from build123d import *

# Parameters (mm, degrees)
AUFSATZ_LINEAR_AUSTRAGEN1_DEPTH = 5
DURCHGANGSLOCH_F_R_M41_D        = 4.3
DURCHGANGSLOCH_F_R_M42_D        = 4.3
M4_GEWINDEBOHRUNG1_D            = 3.3
M3_GEWINDEBOHRUNG1_D            = 2.5


with BuildPart() as part:
    # Skizze1 → Aufsatz-Linear austragen1 (new body)
    with BuildSketch(Plane(origin=(0, 0, 0), x_dir=(1, 0, 0), z_dir=(0, 1, 0))):
        Polygon((-9, 15), (-9, -15), (29, -15), (29, 35), (9, 35), (9, 15), align=None)
    extrude(amount=AUFSATZ_LINEAR_AUSTRAGEN1_DEPTH)

    # Durchgangsloch für M41 (through all)
    with Locations(Plane(origin=(0, 5, 0), x_dir=(1, 0, 0), z_dir=(0, 1, 0))):
        with Locations((7, 8), (23, 8), (7, -8), (23, -8)):
            Hole(DURCHGANGSLOCH_F_R_M41_D / 2)

    # Durchgangsloch für M42 (through all)
    with Locations(Plane(origin=(0, 5, 0), x_dir=(1, 0, 0), z_dir=(0, 1, 0))):
        with Locations((-3.5, 8), (-3.5, -8)):
            Hole(DURCHGANGSLOCH_F_R_M42_D / 2)

    # M4 Gewindebohrung1 (through all)
    with Locations(Plane(origin=(0, 5, 0), x_dir=(1, 0, 0), z_dir=(0, 1, 0))):
        with Locations((19, 25)):
            Hole(M4_GEWINDEBOHRUNG1_D / 2)

    # M3 Gewindebohrung1 (through all)
    with Locations(Plane(origin=(0, 5, 0), x_dir=(1, 0, 0), z_dir=(0, 1, 0))):
        with Locations((3, 0)):
            Hole(M3_GEWINDEBOHRUNG1_D / 2)


solid = part.part
Source: CAD feature listing. Evaluate the final solid. Frame: model axes, mm. A direction names the side the tool comes from. Round coordinates to 2 decimals unless told otherwise and drop trailing zeros. Loops run counter-clockwise (first coordinate to the right, second up) from the corner with the lowest first, then second, coordinate; pieces in that order, holes last.
Q1. Section A-A, the plane x = 23. Return loops of the section in (y, z), plus the area to 3 significant figures.
Q2. Mould query, pull axis Z, two halves, no side actions, for faces 3 (the face through (19, 2, -35)), 4 (the face through (10, 2, 15)), 5 (the face through (9, 2, -25)), 6 (the face through (7.28, 2.47, 5.87)). Classes: pulls with the +Z half, pulls with the -Z half, needs draft (parallel to the pull), parting line crosses it, or undercut.
Q3. Ray query, line 1 (Z direction, x = 23, y = 3.1); line 2 (Z direction, x = 7, y = 4.05); line 3 (X direction, y = 3.4, z = 8). Return the intervals inside material, ascending.
Q4. First-contact query: P1, Ø2.5, axis at x = 2, y = 3.5, coming from the -Z side. Flat tip, straight axial feed; report the tip coordinate or a pass-through.
Q5. Section D-D, the plane z = -25. Return loops of the section in (x, y).
Q6. Section C-C, the plane x = 3. Return loops of the section in (y, z), plus the area to 4 significant figures.
Q7. Section B-B, the plane z = 8. Return loops of the section in (x, y), plus the area to 4 significant figures.
Q8. Access query for faces 1 (the face through (1.81, 2.47, -0.38)), 2 (the face through (0, 2, -15)). Directions: +Z, -Z, +X, -X, +Y, -Y. A direction counts if a zero-diameter tool reaches every point of the face in a straight line with its end or side. Return the directions, or none.
Solutions:
1. outline: (0, -35) - (5, -35) - (5, -10.15) - (0, -10.15) - close; (0, -5.85) - (5, -5.85) - (5, 5.85) - (0, 5.85) - close; (0, 10.15) - (5, 10.15) - (5, 15) - (0, 15) - close
1. area: 207 mm2
2. face 3: pulls with the -Z half
2. face 4: pulls with the +Z half
2. face 5: needs draft
2. face 6: undercut
3. line 1: z = -35 to -10.15, -5.85 to 5.85, 10.15 to 15
3. line 2: z = -15 to -10.15, -5.85 to 5.85, 10.15 to 15
3. line 3: x = -9 to -5.65, -1.35 to 4.85, 9.15 to 20.85, 25.15 to 29
4. P1: stops at z = -15
5. outline: (9, 0) - (17.35, 0) - (17.35, 5) - (9, 5) - close; (20.65, 0) - (29, 0) - (29, 5) - (20.65, 5) - close
6. outline: (0, -15) - (5, -15) - (5, -1.25) - (0, -1.25) - close; (0, 1.25) - (5, 1.25) - (5, 15) - (0, 15) - close
6. area: 137.5 mm2
7. outline: (-9, 0) - (-5.65, 0) - (-5.65, 5) - (-9, 5) - close; (-1.35, 0) - (4.85, 0) - (4.85, 5) - (-1.35, 5) - close; (9.15, 0) - (20.85, 0) - (20.85, 5) - (9.15, 5) - close; (25.15, 0) - (29, 0) - (29, 5) - (25.15, 5) - close
7. area: 125.5 mm2
8. face 1: +Y, -Y
8. face 2: -Z, -X, +Y, -Y
